Geometry check sheet. Reference: drawing and pictorial views, mm from the part's lowest x, y, z. A direction names the side the tool comes from. Give positions to 0.01 mm unless a question says otherwise; leave off trailing zeros. Order: outer loops, then holes, each group sorted by start corner. A loop starts at its lowest first (then second) coordinate and runs counter-clockwise, first axis right, second up.
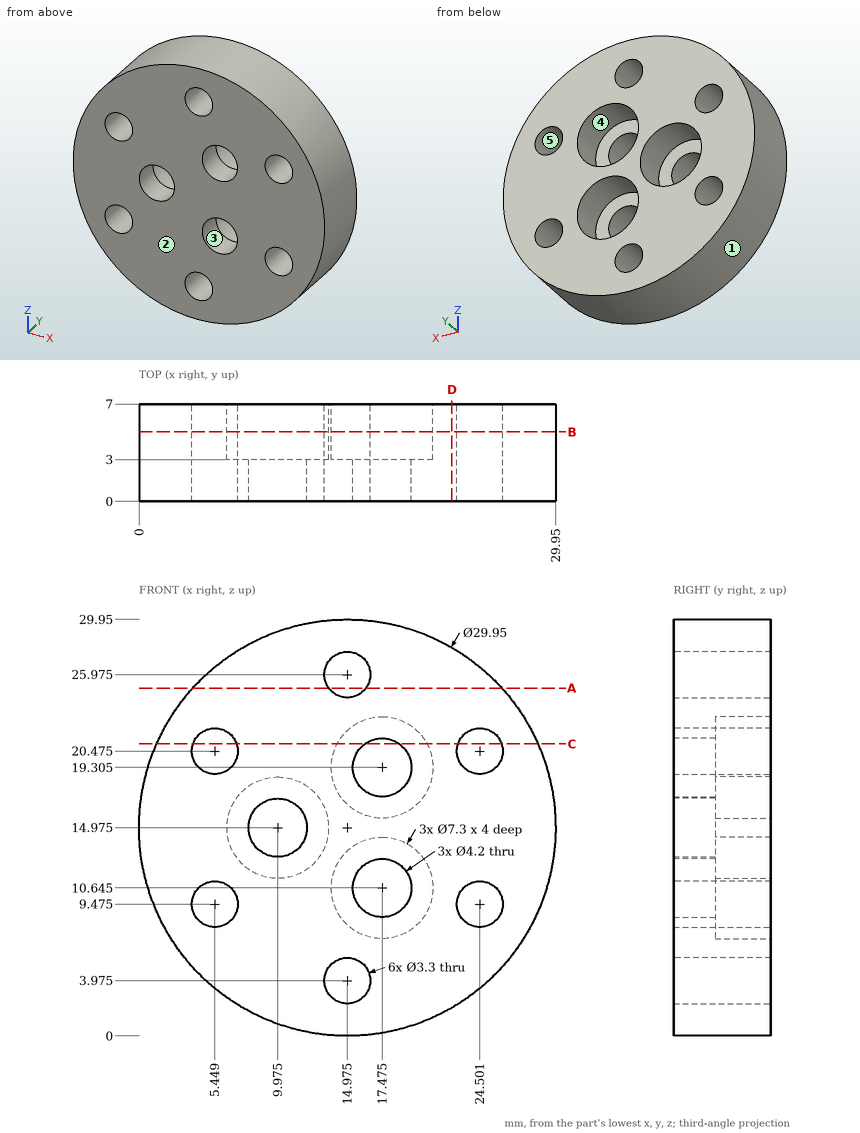
(1) Release check for a two-part mould opening along X. For the marked faces 1, 2 and 3 record: released by +X, released by -X, zero draft, split by the parting line, or undercut.
Response values:
face 1: split by the parting line
face 2: zero draft
face 3: undercut
(2) Set-up check for the marked faces 4 and 5: record each of +Z, -Z, +X, -X, +Y, -Y from which the full face is reachable in a straight line by a thin tool's end or side.
Response values:
face 4: +Y
face 5: +Y, -Y
(3) Material ranges on L1, parallel to X at y = 3.75, z = 13 (1 decimal); L2, parallel to Z at x = 14.25, y = 5.75 (1 decimal); L3, parallel to X at y = 4, z = 18 (1 decimal), recorded low to high.
Response values:
L1: x = 0.1 to 6.9, 13 to 14.7, 20.3 to 29.8
L2: z = 0 to 2.5, 5.5 to 8.9, 12.4 to 17.6, 21 to 24.5, 27.5 to 29.9
L3: x = 0.3 to 7.9, 12 to 14.1, 20.9 to 29.6
(4) Cross-section at D-D on x = 22.5. Enter the section's corners in (y, z).
Response values:
outline: (0, 2.03) - (7, 2.03) - (7, 27.92) - (0, 27.92) - close
(5) Cross-section at C-C on z = 21. Enter the section's corners in (x, y) (1 decimal).
Response values:
outline: (1.3, 0) - (3.9, 0) - (3.9, 7) - (1.3, 7) - close; (7, 0) - (16.2, 0) - (16.2, 3) - (14.2, 3) - (14.2, 7) - (7, 7) - close; (18.7, 0) - (22.9, 0) - (22.9, 7) - (20.7, 7) - (20.7, 3) - (18.7, 3) - close; (26.1, 0) - (28.7, 0) - (28.7, 7) - (26.1, 7) - close
(6) Cross-section at A-A on z = 25. Enter the section's corners in (x, y).
Response values:
outline: (3.85, 0) - (13.64, 0) - (13.64, 7) - (3.85, 7) - close; (16.31, 0) - (26.1, 0) - (26.1, 7) - (16.31, 7) - close
(7) Gauge pin test, flat ends, axial feed: pin 1 Ø1.5 at (x, z) = (15, 18) entering from +Y; pin 2 Ø1 at (y, z) = (4.5, 20.5) entering from -X. Record the tip position at first contact, or that the pin passes through.
Response values:
pin 1: stops at y = 3
pin 2: stops at x = 0.87
(8) Cross-section at B-B on y = 5. Count the separate pieces of the cut face and the enclosed holes in it.
Response values:
separate pieces: 1
enclosed holes: 9
